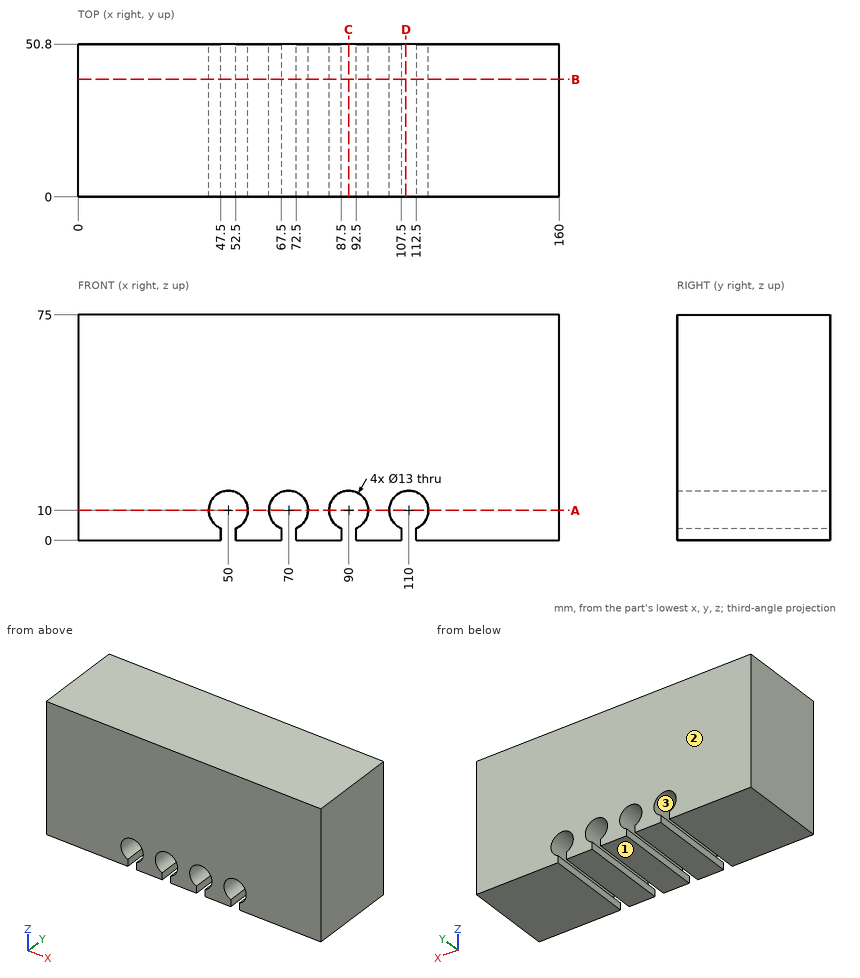
Could you check a few things on this drawing? It's one solid part, dimensions in mm from its lowest x, y, z. Coordinates: 2 decimals unless noted, no trailing zeros. Loops run counter-clockwise (first coordinate to the right, second up) from the corner with the lowest first, then second, coordinate; pieces in that order, holes last.
1. I need wall thicknesses on L1, parallel to X at y = 17, z = 10; L2, parallel to Z at x = 74.5, y = 6; L3, parallel to Z at x = 70, y = 20.5. Which ranges of each line are inside material? Lowest first, please.
2. Imagine slicing it at B-B (y = 39). Please give me the cut outline in (x, z).
3. Imagine slicing it at D-D (x = 109). Please give me the cut outline in (y, z), and give its area (3 significant figures).
4. Imagine slicing it at C-C (x = 90). Please give me the cut outline in (y, z), and give its area (3 significant figures).
5. Imagine slicing it at A-A (z = 10). Please give me the cut outline in (x, y), and give its area (3 significant figures).
6. We'd pull the mould along Z, two halves only. Please class the marked faces 1, 2 and 3: released by +Z, released by -Z, zero draft, split by the parting line, or undercut.
7. For P1, Ø10.5, axis at x = 110, z = 10, coming from the +Y side, with a flat end and sliding along its axis, tell me the tip position at first contact or that it passes through.
Computed values:
1. L1: x = 0 to 43.5, 56.5 to 63.5, 76.5 to 83.5, 96.5 to 103.5, 116.5 to 160
1. L2: z = 0 to 5.31, 14.69 to 75
1. L3: z = 16.5 to 75
2. outline: (0, 0) - (47.5, 0) - (47.5, 4) arc R6.5 cw (long way) to (52.5, 4) - (52.5, 0) - (67.5, 0) - (67.5, 4) arc R6.5 cw (long way) to (72.5, 4) - (72.5, 0) - (87.5, 0) - (87.5, 4) arc R6.5 cw (long way) to (92.5, 4) - (92.5, 0) - (107.5, 0) - (107.5, 4) arc R6.5 cw (long way) to (112.5, 4) - (112.5, 0) - (160, 0) - (160, 75) - (0, 75) - close
3. outline: (0, 16.42) - (50.8, 16.42) - (50.8, 75) - (0, 75) - close
3. area: 2,980 mm2
4. outline: (0, 16.5) - (50.8, 16.5) - (50.8, 75) - (0, 75) - close
4. area: 2,970 mm2
5. outline: (0, 0) - (43.5, 0) - (43.5, 50.8) - (0, 50.8) - close; (56.5, 0) - (63.5, 0) - (63.5, 50.8) - (56.5, 50.8) - close; (76.5, 0) - (83.5, 0) - (83.5, 50.8) - (76.5, 50.8) - close; (96.5, 0) - (103.5, 0) - (103.5, 50.8) - (96.5, 50.8) - close; (116.5, 0) - (160, 0) - (160, 50.8) - (116.5, 50.8) - close
5. area: 5,490 mm2
6. face 1: released by -Z
6. face 2: zero draft
6. face 3: undercut
7. P1: passes through
